Here's how the part is built. I have some questions about the finished solid (model axes, mm). A direction names the side the tool comes from. Round coordinates to 2 decimals unless told otherwise and drop trailing zeros. Order: outer loops, then holes, each group sorted by start corner. A loop starts at its lowest first (then second) coordinate and runs counter-clockwise, first axis right, second up. Notation, with made-up numbers: (-5, 55.25) -> (30, 55.25) arc R13 cw to (30, 73.25) -> close; hole circle Ø1 at (69, 57). An arc over 180 degrees is marked (long way). Use a Markdown table: item, result. Add a question column.
(1) I want a section at A-A, the plane z = 7.5. Please give me the cut outline in (x, y), then the cut area to 3 significant figures.
(2) I want a section at C-C, the plane z = 21. Please give me the cut outline in (x, y), then the cut area to 3 significant figures.
(3) On a 3-axis mill with a long thin cutter (end or side, diameter ignored), from which of +Z, -Z, +X, -X, +Y, -Y can I reach the whole of each face in a straight line? I mean faces 4 (the face through (-2.6, 1.5, 9.9)), 5 (the face through (1.5, 0.7, 20)). Say none if no direction works.
(4) If I drill on probe 1 along Y at (x, z) = (0, 3.65); probe 2 along Z at (x, y) = (0.5, 2.5); probe 3 along X at (y, z) = (-1.5, 18), over which ranges is the centre line in solid material (lowest first)?
(5) Thinking about a two-plate mould opening in Y: for faces 1 (the face through (1.5, 0, 0)), 2 (the face through (-1.5, 0.07, 22.96)), 3 (the face through (-0.27, -1.22, 3.04)), which applies, pulls with the +Y half, pulls with the -Y half, needs draft (parallel to the pull), parting line crosses it, or undercut?
(6) I want a section at D-D, the plane y = 1.75. Please give me the cut outline in (x, z).
(7) I'm going to push flat-ended pins straight in: P1, Ø3, axis at y = 1, z = 15.5, coming from the -X side; P2, Ø1.5, axis at x = 0, y = 0, coming from the -Z side; P3, Ø1.5, axis at x = 1, z = 22, coming from the +Y side. Where does each tip first touch, or does it pass through?
(8) I want a section at B-B, the plane y = -2. Please give me the cut outline in (x, z).
from build123d import *

# Parameters (mm, degrees)
BOSS_EXTRUDE1_DEPTH       = 20
SKETCH2_R                 = 1.5
BOSS_EXTRUDE2_DEPTH       = 6
M3X0_5_TAPPED_HOLE1_D     = 2.5
M3X0_5_TAPPED_HOLE1_DEPTH = 6
M3X0_5_TAPPED_HOLE1_TIP   = 0.751075774


with BuildPart() as part:
    # Sketch1 → Boss-Extrude1 (new body)
    with BuildSketch(Plane.XY):
        Polygon((-3.464101615, 0), (-1.732050808, -3), (1.732050808, -3), (3.464101615, 0), (1.732050808, 3), (-1.732050808, 3), align=None)
    extrude(amount=BOSS_EXTRUDE1_DEPTH)

    # Sketch2 → Boss-Extrude2 (add)
    with BuildSketch(Plane.XY.offset(20)):
        Circle(SKETCH2_R)
    extrude(amount=BOSS_EXTRUDE2_DEPTH)

    # M3x0.5 Tapped Hole1
    with Locations(Plane(origin=(0, 0, 0), x_dir=(-1, 0, 0), z_dir=(0, 0, -1))):
        with Locations((0, 0)):
            Hole(M3X0_5_TAPPED_HOLE1_D / 2, depth=M3X0_5_TAPPED_HOLE1_DEPTH)
            with Locations((0, 0, -(M3X0_5_TAPPED_HOLE1_DEPTH + M3X0_5_TAPPED_HOLE1_TIP / 2))):  # 118° drill point
                Cone(0, M3X0_5_TAPPED_HOLE1_D / 2, M3X0_5_TAPPED_HOLE1_TIP, mode=Mode.SUBTRACT)


solid = part.part
Taken from the geometry:
| question | item | result |
|---|---|---|
| 1 | outline | (-3.46, 0) -> (-1.73, -3) -> (1.73, -3) -> (3.46, 0) -> (1.73, 3) -> (-1.73, 3) -> close |
| 1 | area | 31.2 mm2 |
| 2 | outline | circle Ø3 at (0, 0) |
| 2 | area | 7.07 mm2 |
| 3 | face 4 | +Z, -Z, -X, +Y |
| 3 | face 5 | +Z |
| 4 | probe 1 | y = -3 to -1.25, 1.25 to 3 |
| 4 | probe 2 | z = 0 to 20 |
| 4 | probe 3 | x = -2.6 to 2.6 |
| 5 | face 1 | needs draft |
| 5 | face 2 | parting line crosses it |
| 5 | face 3 | undercut |
| 6 | outline | (-2.45, 0) -> (2.45, 0) -> (2.45, 20) -> (-2.45, 20) -> close |
| 7 | P1 | stops at x = -3.46 |
| 7 | P2 | stops at z = 6.3 |
| 7 | P3 | stops at y = 1.48 |
| 8 | outline | (-2.31, 0) -> (2.31, 0) -> (2.31, 20) -> (-2.31, 20) -> close |
